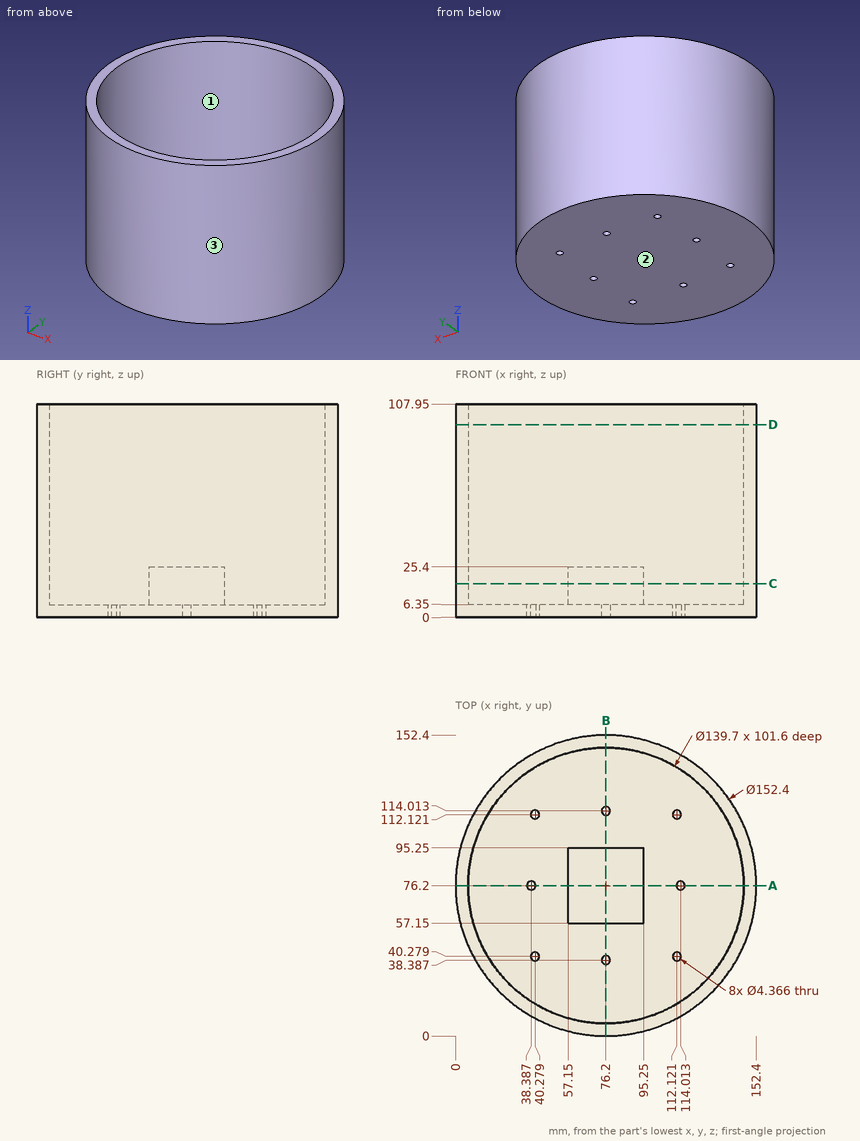
Geometry check sheet. Reference: drawing and pictorial views, mm from the part's lowest x, y, z. Give positions to 0.01 mm unless a question says otherwise; leave off trailing zeros. Loops run counter-clockwise (first coordinate to the right, second up) from the corner with the lowest first, then second, coordinate; pieces in that order, holes last. Notation, with made-up numbers: M 31,76 L 38,76 A14 ccw 38,101 Z; hole C -2.5,68.25 d7. An arc over 180 degrees is marked long. One line per question, with ' | ' between items.
Item 1: Section check A-A, the plane y = 76.2. Record the cut outline in (x, z).
Completed:
outline: M 0,0 L 36.2,0 L 36.2,6.35 L 6.35,6.35 L 6.35,107.95 L 0,107.95 Z; M 40.57,0 L 111.83,0 L 111.83,6.35 L 95.25,6.35 L 95.25,25.4 L 57.15,25.4 L 57.15,6.35 L 40.57,6.35 Z; M 116.2,0 L 152.4,0 L 152.4,107.95 L 146.05,107.95 L 146.05,6.35 L 116.2,6.35 Z
Item 2: Draft check along Y on the marked faces 1, 2 and 3. Enter one of: +Y half, -Y half, draft (parallel to the pull), parting line (faces both ways), or undercut.
Completed:
face 1: undercut | face 2: draft | face 3: parting line
Item 3: Section check D-D, the plane z = 97.5. Record the cut outline in (x, y), plus the area to 3 significant figures.
Completed:
outline: C 76.2,76.2 d152.4; hole C 76.2,76.2 d139.7 | area: 2,910 mm^2
Item 4: Thickness scan on line 1 (Y direction, x = 76.2, z = 3.25); line 2 (Y direction, x = 69, z = 18); line 3 (Z direction, x = 134, y = 115). Record the ranges inside material, lowest first. Write a range as [from, to].
Completed:
line 1: y = [0, 36.2], [40.57, 111.83], [116.2, 152.4] | line 2: y = [0.34, 6.72], [57.15, 95.25], [145.68, 152.06] | line 3: z = [0, 6.35]
Item 5: Depth check by flat-ended pin: P1, Ø6, axis at y = 135.5, z = 68.5, coming from the -X side; P2, Ø10, axis at x = 43, y = 32, coming from the +Z side; P3, Ø11.5, axis at x = 77.5, y = 72, coming from the +Z side; P4, Ø3.5, axis at x = 112.12, y = 40.28, coming from the -Z side. Enter the tip coordinate at first touch or a pass-through.
Completed:
P1: stops at x = 24.85 | P2: stops at z = 6.35 | P3: stops at z = 25.4 | P4: passes through
Item 6: Section check C-C, the plane z = 17. Record the cut outline in (x, y).
Completed:
outline: C 76.2,76.2 d152.4; M 57.15,57.15 L 95.25,57.15 L 95.25,95.25 L 57.15,95.25 Z; hole C 76.2,76.2 d139.7
